The listing builds one solid part. Answer for the finished solid, in the listing's coordinates (mm). Face numbers are marked on the shaded views. Give positions to 0.01 mm unless a question says otherwise; leave off trailing zeros. Order: outer loops, then holes, each group sorted by start corner. A loop starts at its lowest first (then second) coordinate and runs counter-clockwise, first axis right, second up. Notation, with made-up numbers: (-38.75, 44.5) - (-23.75, 44.5) arc R27 cw to (-23.75, 66.5) - close; hole circle Ø5 at (86.25, 14.25). An arc over 180 degrees is marked (long way). Use CSV: the item, a comma, the result in double quotes.
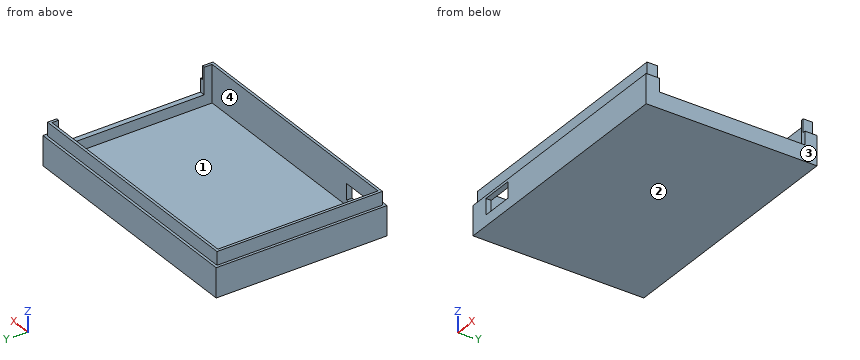
```python
from build123d import *

# Parameters (mm, degrees)
SKETCH1_W           = 94
SKETCH1_H           = 64
BOSS_EXTRUDE1_DEPTH = 16
SKETCH2_W           = 90
SKETCH2_H           = 60
CUT_EXTRUDE1_DEPTH  = 14
SKETCH4_W           = 94
SKETCH4_H           = 64
SKETCH4_W_2         = 92
SKETCH4_H_2         = 62
CUT_EXTRUDE2_DEPTH  = 5
CUT_EXTRUDE3_REACH  = 83
SKETCH6_W           = 12
SKETCH6_H           = 6
CUT_EXTRUDE4_REACH  = 100.712
SKETCH8_W           = 10
SKETCH8_H           = 54.5


with BuildPart() as part:
    # Sketch1 → Boss-Extrude1 (new body)
    with BuildSketch(Plane.XY):
        Rectangle(SKETCH1_W, SKETCH1_H)
    extrude(amount=BOSS_EXTRUDE1_DEPTH)

    # Sketch2 → Cut-Extrude1 (cut)
    with BuildSketch(Plane.XY.offset(16)):
        Rectangle(SKETCH2_W, SKETCH2_H)
    extrude(amount=-CUT_EXTRUDE1_DEPTH, mode=Mode.SUBTRACT)

    # Sketch4 → Cut-Extrude2 (cut)
    with BuildSketch(Plane.XY.offset(16)):
        Rectangle(SKETCH4_W, SKETCH4_H)
        Rectangle(SKETCH4_W_2, SKETCH4_H_2, mode=Mode.SUBTRACT)
    extrude(amount=-CUT_EXTRUDE2_DEPTH, mode=Mode.SUBTRACT)

    # Sketch6 → Cut-Extrude3 (cut, up to next)
    with BuildSketch(Plane.XZ.offset(32), mode=Mode.PRIVATE) as cut_extrude3_sk1:
        with Locations((-34, 7)):
            Rectangle(SKETCH6_W, SKETCH6_H)
    cut_extrude3_tool1 = extrude(cut_extrude3_sk1.sketch, amount=-CUT_EXTRUDE3_REACH, mode=Mode.PRIVATE) & part.part
    add(cut_extrude3_tool1.solids().sort_by_distance((-34, -32, 7))[0], mode=Mode.SUBTRACT)

    # Sketch8 → Cut-Extrude4 (cut, up to next)
    with BuildSketch(Plane.ZY.offset(-45), mode=Mode.PRIVATE) as cut_extrude4_sk1:
        with Locations((11, 0.25)):
            Rectangle(SKETCH8_W, SKETCH8_H)
    cut_extrude4_tool1 = extrude(cut_extrude4_sk1.sketch, amount=-CUT_EXTRUDE4_REACH, mode=Mode.PRIVATE) & part.part
    add(cut_extrude4_tool1.solids().sort_by_distance((45, 0.25, 11))[0], mode=Mode.SUBTRACT)


solid = part.part
```
Item 1: The part is cut by section A-A (z = 8.5). Give the vertices of the cut face in (x, y), and give its area (3 significant figures).
Taken from the geometry:
outline,"(-47, -32) - (-40, -32) - (-40, -30) - (-45, -30) - (-45, 30) - (45, 30) - (45, 27.5) - (47, 27.5) - (47, 32) - (-47, 32) - close; (-28, -32) - (47, -32) - (47, -27) - (45, -27) - (45, -30) - (-28, -30) - close"
area,"483 mm^2"
Item 2: Each of these flat-tipped pins is pushed along its axis until it touches: pin 1 (5.5 mm diameter, centred on x = 21.5, z = 13.5, fed in from +Y); pin 2 (8 mm diameter, centred on x = -20, y = -10.5, fed in from +Z); pin 3 (0.6 mm diameter, centred on x = 46, y = 5, fed in from +Z); pin 4 (1.5 mm diameter, centred on x = -0.5, z = 13.5, fed in from -Y). Where does it stop, or does it pass through?
Taken from the geometry:
pin 1,"y = 32"
pin 2,"z = 2"
pin 3,"z = 6"
pin 4,"y = -31"
Item 3: The part is cut by section C-C (x = -6). Give the vertices of the cut face in (y, z).
Taken from the geometry:
outline,"(-32, 0) - (32, 0) - (32, 11) - (31, 11) - (31, 16) - (30, 16) - (30, 2) - (-30, 2) - (-30, 16) - (-31, 16) - (-31, 11) - (-32, 11) - close"
Item 4: The mould has two halves that part along X. Classify the marked faces 1, 2, 3 and 4: +X half, -X half, draft (parallel to the pull), parting line (faces both ways), or undercut.
Taken from the geometry:
face 1,"undercut"
face 2,"draft"
face 3,"+X half"
face 4,"undercut"
Item 5: Find the intervals of material crossed by line 1 along Y through (x, z) = (-35, 3.5); line 2 along Y through (x, z) = (41.5, 13.5); line 3 along X through (y, z) = (-12, 3), in increasing order.
Taken from the geometry:
line 1,"-32 to -30, 30 to 32"
line 2,"-31 to -30, 30 to 31"
line 3,"-47 to -45, 45 to 47"
Item 6: The part is cut by section B-B (y = -13). Give the vertices of the cut face in (x, z), and give its area (3 significant figures).
Taken from the geometry:
outline,"(-47, 0) - (47, 0) - (47, 6) - (45, 6) - (45, 2) - (-45, 2) - (-45, 16) - (-46, 16) - (-46, 11) - (-47, 11) - close"
area,"219 mm^2"
